Verification items for the finished model (mm, model axes). Coordinates: 2 decimals unless noted, no trailing zeros. Order: outer loops, then holes, each group sorted by start corner. A loop starts at its lowest first (then second) coordinate and runs counter-clockwise, first axis right, second up.
Q1. Depth check by flat-ended pin: P1, Ø3, axis at x = -3.5, z = 4, coming from the -Y side. Enter the tip coordinate at first touch or a pass-through.
Q2. Thickness scan on line 1 (Y direction, x = 5, z = 3); line 2 (X direction, y = -18, z = 1.25); line 3 (Y direction, x = -2, z = 2). Record the ranges inside material, lowest first.
Q3. Cross-section at D-D, the plane y = -34.5. Record the boundary of the cut face in (x, z).
Q4. Cross-section at B-B, the plane z = 4. Record the boundary of the cut face in (x, y), and give its area (3 significant figures).
Q5. Cross-section at A-A, the plane y = -6.5. Record the boundary of the cut face in (x, z).
Q6. Cross-section at C-C, the plane x = -58.5. Record the boundary of the cut face in (y, z), and give its area (3 significant figures).
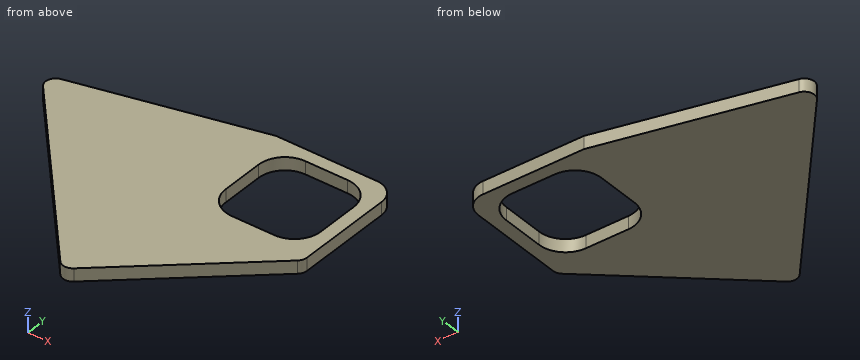
from build123d import *

# Parameters (mm, degrees)
BOSS_EXTRUDE1_DEPTH = 6.35
FILLET1_R           = 10
FILLET2_R           = 5
CUT_EXTRUDE1_DEPTH  = 7.35


with BuildPart() as part:
    # Sketch2 → Boss-Extrude1 (new body)
    with BuildSketch(Plane.XY):
        Polygon((-30, 30), (30, 30), (30, -30), (-41.471442061, -92.584606492), (-128.09675639, 7.014865983), align=None)
    extrude(amount=BOSS_EXTRUDE1_DEPTH)

    # Fillet1
    fillet1_edges = [part.edges().sort_by_distance(p)[0] for p in [
        (30, 30, 3.175),
    ]]
    fillet(fillet1_edges, radius=FILLET1_R)

    # Fillet2
    fillet2_edges = [part.edges().sort_by_distance(p)[0] for p in [
        (-41.471442061, -92.584606492, 3.175),
        (-128.09675639, 7.014865983, 3.175),
        (30, -30, 3.175),
    ]]
    fillet(fillet2_edges, radius=FILLET2_R)

    # Sketch3 → Cut-Extrude1 (cut, through all)
    with BuildSketch(Plane.XY.offset(6.35)):
        with BuildLine():
            Line((-10.5, 23.5), (10.5, 23.5))
            ThreePointArc((10.5, 23.5), (19.692388155, 19.692388155), (23.5, 10.5))
            Line((23.5, 10.5), (23.5, -10.5))
            ThreePointArc((23.5, -10.5), (19.692388155, -19.692388155), (10.5, -23.5))
            Line((10.5, -23.5), (-10.5, -23.5))
            ThreePointArc((-10.5, -23.5), (-19.692388155, -19.692388155), (-23.5, -10.5))
            Line((-23.5, -10.5), (-23.5, 10.5))
            ThreePointArc((-23.5, 10.5), (-19.692388155, 19.692388155), (-10.5, 23.5))
        make_face()
    extrude(amount=-CUT_EXTRUDE1_DEPTH, mode=Mode.SUBTRACT)


solid = part.part
Check values:
1. P1: stops at y = -60.65
2. line 1: y = -51.89 to -23.5, 23.5 to 30
2. line 2: x = -106.34 to -21.12, 21.12 to 30
2. line 3: y = -58.02 to -23.5, 23.5 to 30
3. outline: (-91.99, 0) - (24.86, 0) - (24.86, 6.35) - (-91.99, 6.35) - close
4. outline: (-122.65, 0.76) - (-44.76, -88.8) arc R5 ccw to (-37.7, -89.28) - (28.29, -31.49) arc R5 ccw to (30, -27.73) - (30, 20) arc R10 ccw to (20, 30) - (-30, 30) - (-120.02, 8.91) arc R5 ccw to start; hole (-23.5, -10.5) arc R13 ccw to (-10.5, -23.5) - (10.5, -23.5) arc R13 ccw to (23.5, -10.5) - (23.5, 10.5) arc R13 ccw to (10.5, 23.5) - (-10.5, 23.5) arc R13 ccw to (-23.5, 10.5) - close
4. area: 9,600 mm2
5. outline: (-116.34, 0) - (-23.5, 0) - (-23.5, 6.35) - (-116.34, 6.35) - close; (23.5, 0) - (30, 0) - (30, 6.35) - (23.5, 6.35) - close
6. outline: (-73.01, 0) - (23.32, 0) - (23.32, 6.35) - (-73.01, 6.35) - close
6. area: 612 mm2
